from build123d import *

# Parameters (mm, degrees)
BOSS_EXTRUDE1_START   = -24
BOSS_EXTRUDE1_DEPTH   = 4
BOSS_EXTRUDE1_START_2 = 20
BOSS_EXTRUDE1_2_DEPTH = 4
SKETCH3_W             = 48
SKETCH3_H             = 150.572975632
BOSS_EXTRUDE2_DEPTH   = 4
SKETCH4_W             = 87.955919885
SKETCH4_H             = 41.238898543
CUT_EXTRUDE1_DEPTH    = 10
CHAMFER1_SIZE         = 5
CHAMFER2_SIZE         = 7
CUT_EXTRUDE2_DEPTH    = 100
BOSS_EXTRUDE3_REACH   = 158.663
SKETCH7_R             = 1.6
BOSS_EXTRUDE4_DEPTH   = 3
CUT_EXTRUDE3_DEPTH    = 13


# Read off the part's stored shape, not the designer's step: Boss-Extrude1
with BuildPart() as part:
    # Boss-Extrude1 outline → Boss-Extrude1 (new body)
    with BuildSketch(Plane.YZ.offset(BOSS_EXTRUDE1_START)):
        Polygon((-230, 56.247033646), (-230, 0), (-80, 0), (-80, 43.123734117), align=None)
    extrude(amount=BOSS_EXTRUDE1_DEPTH)



with BuildPart() as body_2:
    # Boss-Extrude1 2 outline → Boss-Extrude1 2 (new body)
    with BuildSketch(Plane.YZ.offset(BOSS_EXTRUDE1_START_2)):
        Polygon((-230, 56.247033646), (-230, 0), (-80, 0), (-80, 43.123734117), align=None)
    extrude(amount=BOSS_EXTRUDE1_2_DEPTH)


with BuildPart() as part_1:
    add(part.part)

    add(body_2.part)  # Boss-Extrude2 merges body 2
    # Sketch3 → Boss-Extrude2 (add)
    with BuildSketch(Plane(origin=(0, 3.136489042, 35.850233801), x_dir=(1, 0, 0), z_dir=(-5.546132053355945e-15, 0.08715574274765837, 0.9961946980917457))):
        with Locations((0, -158.74054474)):
            Rectangle(SKETCH3_W, SKETCH3_H)
    extrude(amount=-BOSS_EXTRUDE2_DEPTH)

    # Sketch4 → Cut-Extrude1 (cut)
    with BuildSketch(Plane.XZ.offset(230)):
        with Locations((0.013546112, 51.627258861)):
            Rectangle(SKETCH4_W, SKETCH4_H)
    extrude(amount=CUT_EXTRUDE1_DEPTH, mode=Mode.SUBTRACT)

    # Chamfer1
    chamfer1_edges = [part_1.edges().sort_by_distance(p)[0] for p in [
        (-20, -155.174311485, 45.685354811),
        (20, -155.174311485, 45.685354811),
    ]]
    chamfer(chamfer1_edges, length=CHAMFER1_SIZE)

    # Chamfer2
    # the kernel refuses this chamfer: 7 mm, written as the material it takes off along each edge
    with BuildSketch(Plane(origin=(24, -62.066721296, 41.55477553), x_dir=(0.027495876610592048, -0.08712279063597585, -0.9958180537232768), z_dir=(0, -0.9961946980916814, 0.0871557427483924)), Plane(origin=(-24, -62.066721296, 41.55477553), x_dir=(0.9996219169112968, 0.0023964235485137053, 0.027391246498848068), z_dir=(0, -0.9961946980916814, 0.0871557427483924))) as chamfer2_piece_1:
        Polygon((CHAMFER2_SIZE * 0.999621916911, -CHAMFER2_SIZE * 0.0274958766106), (-CHAMFER2_SIZE * 0.0274958766106, -CHAMFER2_SIZE * 0.999621916911), (0, 0), align=None)
    extrude(amount=186.576537463, mode=Mode.SUBTRACT)

    # Sketch5 → Cut-Extrude2 (cut)
    with BuildSketch(Plane.ZY.offset(24)):
        with BuildLine():
            Line((27.989036278, -104.58131235), (33.229814206, -204.58131235))
            ThreePointArc((33.229814206, -204.58131235), (25.659465578, -212.989036278), (17.25174165, -205.41868765))
            Line((17.25174165, -205.41868765), (12.010963722, -105.41868765))
            ThreePointArc((12.010963722, -105.41868765), (19.58131235, -97.010963722), (27.989036278, -104.58131235))
        make_face()
    extrude(amount=-CUT_EXTRUDE2_DEPTH, mode=Mode.SUBTRACT)

    # Boss-Extrude3: up to this face of the body (flat: up to its plane)
    boss_extrude3_end = Plane(part_1.part.faces().sort_by_distance((21.96487497, -80, 19.069947066))[0])
    # Sketch6 → Boss-Extrude3 (add, up to the picked face)
    with BuildSketch(Plane(origin=(0, -83.136489042, 7.273500317), x_dir=(1, 0, 0), z_dir=(0, 0.9961946980917457, -0.0871557427476584)), mode=Mode.PRIVATE) as boss_extrude3_sk1:
        Polygon((20, -32.98717587), (20, -26.98717587), (15, -31.98717587), (-15, -31.98717587), (-20, -26.98717587), (-20, -32.98717587), (-17, -35.98717587), (17, -35.98717587), align=None)
    boss_extrude3_tool1 = split(extrude(boss_extrude3_sk1.sketch, amount=BOSS_EXTRUDE3_REACH, mode=Mode.PRIVATE), bisect_by=boss_extrude3_end, keep=Keep.BOTH, mode=Mode.PRIVATE)
    add(boss_extrude3_tool1.solids().sort_by(Axis((0, -80.224162, 40.561552), (0, 0.9961946980917457, -0.0871557427476584)))[0])

    # Sketch7 → Boss-Extrude4 (add)
    # profile 1 of 4: a face of its own
    with BuildSketch(Plane(origin=(0, 0, 0), x_dir=(-1, 0, 0), z_dir=(0, 0, -1))):
        Polygon((-24, -80), (-32, -84.618802154), (-32, -94.618802154), (-24, -99.237604307), align=None)
        with Locations((-28, -89.618802154)):
            Circle(SKETCH7_R, mode=Mode.SUBTRACT)
    # profile 2 of 4: a face of its own
    with BuildSketch(Plane(origin=(0, 0, 0), x_dir=(-1, 0, 0), z_dir=(0, 0, -1))):
        Polygon((-24, -210.762395693), (-24, -230), (-32, -225.381197846), (-32, -215.381197846), align=None)
        with Locations(Location((-28, -220.381197846, 0), (0, 0, 180))):
            Circle(SKETCH7_R, mode=Mode.SUBTRACT)
    # profile 3 of 4: a face of its own
    with BuildSketch(Plane(origin=(0, 0, 0), x_dir=(-1, 0, 0), z_dir=(0, 0, -1))):
        Polygon((24, -230), (32, -225.381197846), (32, -215.381197846), (24, -210.762395693), align=None)
        with Locations((28, -220.381197846)):
            Circle(SKETCH7_R, mode=Mode.SUBTRACT)
    # profile 4 of 4: a face of its own
    with BuildSketch(Plane(origin=(0, 0, 0), x_dir=(-1, 0, 0), z_dir=(0, 0, -1))):
        Polygon((24, -99.237604307), (24, -80), (32, -84.618802154), (32, -94.618802154), align=None)
        with Locations(Location((28, -89.618802154, 0), (0, 0, 180))):
            Circle(SKETCH7_R, mode=Mode.SUBTRACT)
    extrude(amount=-BOSS_EXTRUDE4_DEPTH)

    # Sketch8 → Cut-Extrude3 (cut)
    with BuildSketch(Plane(origin=(0, 3.136489042, 35.850233801), x_dir=(1, 0, 0), z_dir=(-5.546132053355945e-15, 0.08715574274765837, 0.9961946980917457))):
        with BuildLine():
            Line((8, -108.454056924), (8, -209.027032556))
            ThreePointArc((8, -209.027032556), (0, -217.027032556), (-8, -209.027032556))
            Line((-8, -209.027032556), (-8, -108.454056924))
            ThreePointArc((-8, -108.454056924), (0, -100.454056924), (8, -108.454056924))
        make_face()
    extrude(amount=-CUT_EXTRUDE3_DEPTH, mode=Mode.SUBTRACT)


solid = part_1.part
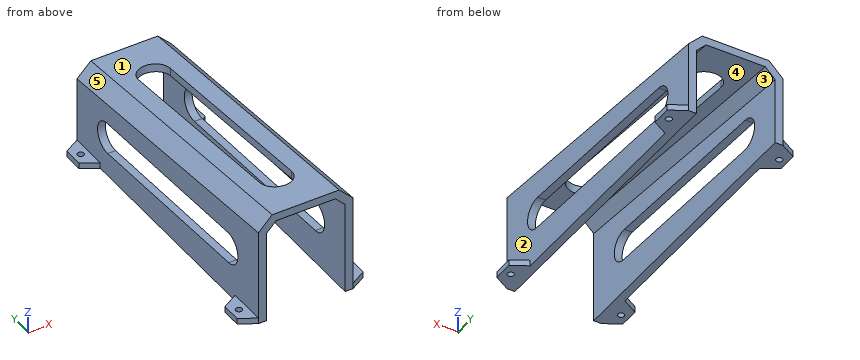
Can you work these out from the model? Positions are in its coordinate system, mm. Face numbers are marked on the shaded views. A direction names the side the tool comes from. Coordinates: 2 decimals unless noted, no trailing zeros. Loops run counter-clockwise (first coordinate to the right, second up) from the corner with the lowest first, then second, coordinate; pieces in that order, holes last. Notation, with made-up numbers: (-7, 40.25) - (30, 40.25) arc R25 cw to (30, 67.25) - close; hole circle Ø7 at (8.5, 70). An arc over 180 degrees is marked (long way). Answer as a JSON object with one key per item and string values. Group by question number.
Item 1: If we section it at D-D (z = 6.5): List the corners of the cut face in (x, y) for me.
Item 2: If we section it at B-B (z = 20): List the corners of the cut face in (x, y) for me.
Item 3: For pin 1 (1 mm diameter, centred on y = -139.5, z = 32.5, fed in from +X); pin 2 (6 mm diameter, centred on x = -19, y = -97, fed in from -Z); pin 3 (1 mm diameter, centred on x = -11, y = -124.5, fed in from -Z); pin 4 (3 mm diameter, centred on x = -12.5, y = -101.5, fed in from -Z), each with a flat end and sliding along its axis, tell me the tip position at first contact or that it passes through.
Item 4: If we mould it in two halves opening along X, with no side actions, what happens to the marked faces 1, 2 and 3? For each: released by +X, released by -X, zero draft, split by the parting line, or undercut.
Item 5: On a 3-axis mill with a long thin cutter (end or side, diameter ignored), from which of +Z, -Z, +X, -X, +Y, -Y can I reach the whole of each face in a straight line? I mean the marked faces 4 and 5. Say none if no direction works.
Item 6: If we section it at A-A (y = -150): List the corners of the cut face in (x, z) for me.
Item 7: If we section it at C-C (x = 6.5): List the corners of the cut face in (y, z) for me, plus the area to 3 significant figures.
Item 8: If I drill on L1, parallel to X at y = -204, z = 37; L2, parallel to Y at x = -28, z = 1.5; L3, parallel to X at y = -200.5, z = 51, over which ranges is the centre line in solid material (lowest first)? Write a range as from..to.
Returned:
{
 "1": {"outline": "(-24, -230) - (-20, -230) - (-20, -80) - (-24, -80) - close; (20, -230) - (24, -230) - (24, -80) - (20, -80) - close"},
 "2": {"outline": "(-24, -230) - (-20, -230) - (-20, -211.04) - (-24, -211.04) - close; (-24, -97) - (-20, -97) - (-20, -80) - (-24, -80) - close; (20, -230) - (24, -230) - (24, -211.04) - (20, -211.04) - close; (20, -97) - (24, -97) - (24, -80) - (20, -80) - close"},
 "3": {"pin 1": "stops at x = 24", "pin 2": "stops at z = 0", "pin 3": "stops at z = 42.96", "pin 4": "stops at z = 40.86"},
 "4": {"face 1": "zero draft", "face 2": "released by +X", "face 3": "undercut"},
 "5": {"face 4": "-Z, -Y", "face 5": "+Z, -X, +Y"},
 "6": {"outline": "(-24, 0) - (-20, 0) - (-20, 14.35) - (-24, 14.35) - close; (-24, 30.37) - (-20, 30.37) - (-20, 40.21) - (-15, 45.23) - (-8, 45.23) - (-8, 49.25) - (-17, 49.25) - (-24, 42.22) - close; (8, 45.23) - (15, 45.23) - (20, 40.21) - (20, 30.37) - (24, 30.37) - (24, 42.22) - (17, 49.25) - (8, 49.25) - close; (20, 0) - (24, 0) - (24, 14.35) - (20, 14.35) - close"},
 "7": {"outline": "(-230, 52.23) - (-210.09, 50.49) - (-209.74, 54.47) - (-230, 56.25) - close; (-100.61, 40.91) - (-80, 39.11) - (-80, 43.12) - (-100.26, 44.9) - close", "area": "163 mm²"},
 "8": {"L1": "x = -24..-20, 20..24", "L2": "y = -227.69..-221.98, -218.78..-213.07, -96.93..-91.22, -88.02..-82.31", "L3": "x = -19.66..-8, 8..19.66"}
}
